from build123d import *

# Parameters (mm, degrees)
SKETCH_3_R          = 73
EXTRUDE_3_DEPTH     = 2.5
SKETCH_5_R          = 67
CUT_EXTRUDE_1_DEPTH = 2.5
SKETCH_6_R          = 15
EXTRUDE_4_DEPTH     = 2.5
SKETCH_7_R          = 8
CUT_EXTRUDE_2_DEPTH = 2.5
EXTRUDE_6_DEPTH     = 2.5
EXTRUDE_7_DEPTH     = 2.5
EXTRUDE_8_DEPTH     = 2.5
EXTRUDE_9_DEPTH     = 2.5
EXTRUDE_10_DEPTH    = 2.5
SKETCH_14_R         = 8
CUT_EXTRUDE_3_DEPTH = 2.5
SKETCH_15_R         = 1
CUT_EXTRUDE_4_DEPTH = 2.5


with BuildPart() as part:
    # Sketch 3 → Extrude 3 (new body)
    with BuildSketch(Plane.XY):
        Circle(SKETCH_3_R)
    extrude(amount=EXTRUDE_3_DEPTH)

    # Sketch 5 → Cut-Extrude 1 (cut)
    with BuildSketch(Plane.XY.offset(2.5)):
        Circle(SKETCH_5_R)
    extrude(amount=-CUT_EXTRUDE_1_DEPTH, mode=Mode.SUBTRACT)



with BuildPart() as body_2:
    # Sketch 6 → Extrude 4 (new body)
    with BuildSketch(Plane.XY.offset(2.5)):
        Circle(SKETCH_6_R)
    extrude(amount=-EXTRUDE_4_DEPTH)

    # Sketch 7 → Cut-Extrude 2 (cut)
    with BuildSketch(Plane.XY.offset(2.5)):
        Circle(SKETCH_7_R)
    extrude(amount=-CUT_EXTRUDE_2_DEPTH, mode=Mode.SUBTRACT)


with BuildPart() as part_1:
    add(part.part)

    add(body_2.part)  # Extrude 6 merges body 2
    # Sketch 9 → Extrude 6 (add)
    with BuildSketch(Plane.XY.offset(2.5)):
        with BuildLine():
            Line((0, 2), (0, 0))
            Line((0, 0), (0, -2))
            Line((0, -2), (66.970142601, -2))
            ThreePointArc((66.970142601, -2), (67, 0), (66.970142601, 2))
            Line((66.970142601, 2), (0, 2))
        make_face()
    extrude(amount=-EXTRUDE_6_DEPTH)

    # Sketch 10 → Extrude 7 (add)
    with BuildSketch(Plane.XY.offset(2.5)):
        with BuildLine():
            Line((1.902113033, -0.618033989), (0, 0))
            Line((0, 0), (-1.902113033, 0.618033989))
            Line((-1.902113033, 0.618033989), (18.792799147, 64.310424507))
            ThreePointArc((18.792799147, 64.310424507), (20.704138623, 63.720786592), (22.597025212, 63.074356529))
            Line((22.597025212, 63.074356529), (1.902113033, -0.618033989))
        make_face()
    extrude(amount=-EXTRUDE_7_DEPTH)

    # Sketch 11 → Extrude 8 (add)
    with BuildSketch(Plane.XY.offset(2.5)):
        with BuildLine():
            Line((0, 0), (1.175570505, 1.618033989))
            Line((1.175570505, 1.618033989), (-53.004412975, 40.982096154))
            ThreePointArc((-53.004412975, 40.982096154), (-54.204138623, 39.381611904), (-55.355553985, 37.746028176))
            Line((-55.355553985, 37.746028176), (-1.175570505, -1.618033989))
            Line((-1.175570505, -1.618033989), (0, 0))
        make_face()
    extrude(amount=-EXTRUDE_8_DEPTH)

    # Sketch 12 → Extrude 9 (add)
    with BuildSketch(Plane.XY.offset(2.5)):
        with BuildLine():
            Line((0, 0), (1.175570505, -1.618033989))
            Line((1.175570505, -1.618033989), (-53.004412975, -40.982096154))
            ThreePointArc((-53.004412975, -40.982096154), (-54.176759621, -39.419268347), (-55.30304181, -37.822923823))
            Line((-55.30304181, -37.822923823), (-1.175570505, 1.618033989))
            Line((-1.175570505, 1.618033989), (0, 0))
        make_face()
    extrude(amount=-EXTRUDE_9_DEPTH)

    # Sketch 13 → Extrude 10 (add)
    with BuildSketch(Plane.XY.offset(2.5)):
        with BuildLine():
            Line((0, 0), (1.902113033, 0.618033989))
            Line((1.902113033, 0.618033989), (22.597025212, -63.074356529))
            ThreePointArc((22.597025212, -63.074356529), (20.704138623, -63.720786592), (18.792799147, -64.310424507))
            Line((18.792799147, -64.310424507), (-1.902113033, -0.618033989))
            Line((-1.902113033, -0.618033989), (0, 0))
        make_face()
    extrude(amount=-EXTRUDE_10_DEPTH)

    # Sketch 14 → Cut-Extrude 3 (cut)
    with BuildSketch(Plane.XY.offset(2.5)):
        Circle(SKETCH_14_R)
    extrude(amount=-CUT_EXTRUDE_3_DEPTH, mode=Mode.SUBTRACT)

    # Sketch 15 → Cut-Extrude 4 (cut)
    with BuildSketch(Plane.XY.offset(2.5)):
        with Locations((70, 0)):
            Circle(SKETCH_15_R)
        with Locations((21.631189606, 66.573956141)):
            Circle(SKETCH_15_R)
        with Locations((-56.631189606, 41.14496766)):
            Circle(SKETCH_15_R)
        with Locations((-56.631189606, -41.14496766)):
            Circle(SKETCH_15_R)
        with Locations((21.631189606, -66.573956141)):
            Circle(SKETCH_15_R)
    extrude(amount=-CUT_EXTRUDE_4_DEPTH, mode=Mode.SUBTRACT)


solid = part_1.part
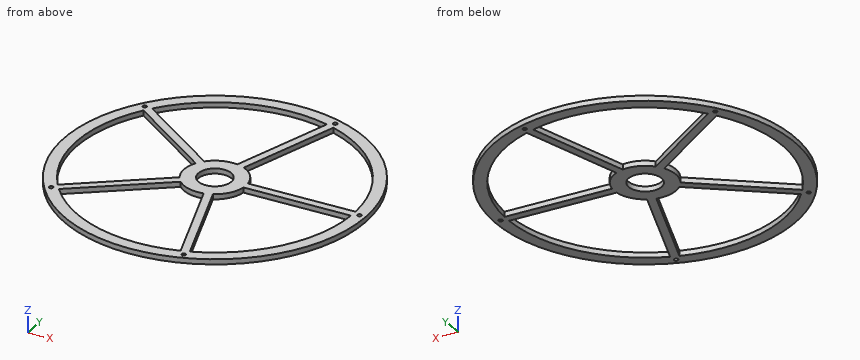
Model file for the job. Use its own axes, mm. Give positions to 0.01 mm unless a question says otherwise; leave off trailing zeros. Order: outer loops, then holes, each group sorted by start corner. A loop starts at its lowest first (then second) coordinate and runs counter-clockwise, first axis right, second up. Notation, with made-up numbers: M 76,22.5 L 134,22.5 A17 ccw 134,38.5 Z; hole C 22.5,37.25 d4. An arc over 180 degrees is marked long. Put each result on its own line as item: value. Start each with the question number.
(1) Band-saw the part on A-A on x = 0. Give the cut face in (y, z).
(2) Band-saw the part on C-C on y = 59. Give the cut face in (x, z), then the cut area to 3 significant figures.
(3) Pin check, flat tips, straight feed: pin 1 Ø1.6 at (x, y) = (-56.63, 41.14) entering from +Z; pin 2 Ø1.5 at (x, z) = (-51, 1.5) entering from +Y; pin 3 Ø1 at (y, z) = (3, 0.5) entering from +X. Stop position of each tip, or through.
(4) Band-saw the part on D-D on z = 0.8. Count the separate pieces of the cut face and the enclosed holes in it, then the cut area to 3 significant figures.
(5) Band-saw the part on B-B on y = -29.5. Give the cut face in (x, z), then the cut area to 3 significant figures.
(6) Drill centre lines: L1, parallel to X at y = -16.5, z = 2.45; L2, parallel to X at y = 46.5, z = 0.75; L3, parallel to Y at x = -6, z = 0.6. Where is each one in solid material? Low to high. Write a range as [from, to].
Results below:
1. outline: M -73,0 L -67,0 L -67,2.5 L -73,2.5 Z; M -15,0 L -8,0 L -8,2.5 L -15,2.5 Z; M 8,0 L 15,0 L 15,2.5 L 8,2.5 Z; M 67,0 L 73,0 L 73,2.5 L 67,2.5 Z
2. outline: M -42.99,0 L -31.75,0 L -31.75,2.5 L -42.99,2.5 Z; M 17.07,0 L 21.27,0 L 21.27,2.5 L 17.07,2.5 Z; M 31.75,0 L 42.99,0 L 42.99,2.5 L 31.75,2.5 Z
2. area: 66.7 mm2
3. pin 1: passes through
3. pin 2: stops at y = 52.95
3. pin 3: stops at x = 72.96
4. separate pieces: 1
4. enclosed holes: 11
4. area: 4,170 mm2
5. outline: M -66.77,0 L -60.16,0 L -60.16,2.5 L -66.77,2.5 Z; M -43.88,0 L -37.2,0 L -37.2,2.5 L -43.88,2.5 Z; M 7.48,0 L 11.69,0 L 11.69,2.5 L 7.48,2.5 Z; M 60.16,0 L 66.77,0 L 66.77,2.5 L 60.16,2.5 Z
5. area: 60.3 mm2
6. L1: x = [-71.11, -64.94], [-26.04, -19.31], [3.26, 7.46], [64.94, 71.11]
6. L2: x = [-56.27, -48.24], [13.01, 17.21], [48.24, 56.27]
6. L3: y = [-72.75, -66.73], [-13.75, -5.29], [5.29, 13.75], [66.73, 72.75]
